Geometry: final body of the model. Coordinates: model frame, mm. A direction names the side the tool comes from. Give positions to 0.01 mm unless a question says otherwise; leave off trailing zeros. Order: outer loops, then holes, each group sorted by start corner. A loop starts at its lowest first (then second) coordinate and runs counter-clockwise, first axis right, second up. Notation, with made-up numbers: (-12.5, 38.5) - (40.5, 38.5) arc R18 cw to (40.5, 64.5) - close; hole circle Ø4 at (48, -35). An arc over 180 degrees is marked (long way). Use one line per item in the form item = value.
from build123d import *

# Parameters (mm, degrees)
F0_R     = 25
F1_DEPTH = 10


# Not quite as in the source:
# - a feature names something its author has since deleted; it is built from what else it names


with BuildPart() as f1:
    # F0 (on Top) → F1 (new body)
    with BuildSketch(Plane.XY):
        with Locations((-0.1409200142, -0.0023476887)):
            Circle(F0_R)
        with BuildLine():
            ThreePointArc((0.7, 23.7306175986), (17.033068856, 16.5380402997), (23.7409395688, 0))
            ThreePointArc((23.7409395688, 0), (23.0200904836, -5.8058286004), (20.9013176879, -11.2590910166))
            ThreePointArc((20.9013176879, -11.2590910166), (20.5602567763, -11.8704697844), (20.2013176879, -12.4715265819))
            ThreePointArc((20.2013176879, -12.4715265819), (0, -23.7409395688), (-20.2013176879, -12.4715265819))
            ThreePointArc((-20.2013176879, -12.4715265819), (-20.5602567763, -11.8704697844), (-20.9013176879, -11.2590910166))
            ThreePointArc((-20.9013176879, -11.2590910166), (-20.5602567763, 11.8704697844), (-0.7, 23.7306175986))
            ThreePointArc((-0.7, 23.7306175986), (0, 23.7409395688), (0.7, 23.7306175986))
        make_face(mode=Mode.SUBTRACT)
        with BuildLine():
            ThreePointArc((5.4607696164, 0), (4.1013743754, 3.6053755749), (0.7, 5.4157183091))
            ThreePointArc((0.7, 5.4157183091), (0.3507241153, 5.4494951508), (0, 5.4607696164))
            ThreePointArc((0, 5.4607696164), (-0.3507241153, 5.4494951508), (-0.7, 5.4157183091))
            ThreePointArc((-0.7, 5.4157183091), (-4.729165212, 2.7303848082), (-5.0401496354, -2.1016413719))
            ThreePointArc((-5.0401496354, -2.1016413719), (-4.8947632961, -2.4210115818), (-4.729165212, -2.7303848082))
            ThreePointArc((-4.729165212, -2.7303848082), (-4.5440391807, -3.028483569), (-4.3401496354, -3.3140769372))
            ThreePointArc((-4.3401496354, -3.3140769372), (0, -5.4607696164), (4.3401496354, -3.3140769372))
            ThreePointArc((4.3401496354, -3.3140769372), (4.5440391807, -3.028483569), (4.729165212, -2.7303848082))
            ThreePointArc((4.729165212, -2.7303848082), (4.8947632961, -2.4210115818), (5.0401496354, -2.1016413719))
            ThreePointArc((5.0401496354, -2.1016413719), (5.354582187, -1.0716596503), (5.4607696164, 0))
        make_face()
        with BuildLine():
            Line((-3.4987264855, 2.0612527399), (0, 2.0612527399))
            Line((0, 2.0612527399), (3.4987264855, 2.0612527399))
            ThreePointArc((3.4987264855, 2.0612527399), (0, -3.5618006487), (-3.4987264855, 2.0612527399))
        make_face(mode=Mode.SUBTRACT)
        with BuildLine():
            Line((-5.0401496354, -2.1016413719), (-20.9013176879, -11.2590910166))
            ThreePointArc((-20.9013176879, -11.2590910166), (-20.5602567763, -11.8704697844), (-20.2013176879, -12.4715265819))
            Line((-20.2013176879, -12.4715265819), (-4.3401496354, -3.3140769372))
            ThreePointArc((-4.3401496354, -3.3140769372), (-4.5440391807, -3.028483569), (-4.729165212, -2.7303848082))
            ThreePointArc((-4.729165212, -2.7303848082), (-4.8947632961, -2.4210115818), (-5.0401496354, -2.1016413719))
        make_face()
        with BuildLine():
            Line((0.7, 5.4157183091), (0.7, 23.7306175986))
            ThreePointArc((0.7, 23.7306175986), (0, 23.7409395688), (-0.7, 23.7306175986))
            Line((-0.7, 23.7306175986), (-0.7, 5.4157183091))
            ThreePointArc((-0.7, 5.4157183091), (-0.3507241153, 5.4494951508), (0, 5.4607696164))
            ThreePointArc((0, 5.4607696164), (0.3507241153, 5.4494951508), (0.7, 5.4157183091))
        make_face()
        with BuildLine():
            ThreePointArc((20.2013176879, -12.4715265819), (20.5602567763, -11.8704697844), (20.9013176879, -11.2590910166))
            Line((20.9013176879, -11.2590910166), (5.0401496354, -2.1016413719))
            ThreePointArc((5.0401496354, -2.1016413719), (4.8947632961, -2.4210115818), (4.729165212, -2.7303848082))
            ThreePointArc((4.729165212, -2.7303848082), (4.5440391807, -3.028483569), (4.3401496354, -3.3140769372))
            Line((4.3401496354, -3.3140769372), (20.2013176879, -12.4715265819))
        make_face()
    extrude(amount=F1_DEPTH)


solid = f1.part
(1) Reachability of faces 1 (the face through (20.39, 12.16, 4.93)), 2 (the face through (0, 4, 10)) from +Z, -Z, +X, -X, +Y, -Y: full face, straight path, thin tool, end or side. Return the list, or none.
Computed values:
face_1 = +Z, -Z
face_2 = +Z, +X, -X, +Y, -Y
(2) Cut plane C-C on y = -14.5. Output: boundary loops of the cut face in (x, z), plus the area to 3 significant figures.
Computed values:
outline = (-20.51, 0) - (-18.8, 0) - (-18.8, 10) - (-20.51, 10) - close; (18.8, 0) - (20.23, 0) - (20.23, 10) - (18.8, 10) - close
area = 31.4 mm²
(3) Cut plane B-B on x = -16. Output: boundary loops of the cut face in (y, z).
Computed values:
outline = (-19.33, 0) - (-17.54, 0) - (-17.54, 10) - (-19.33, 10) - close; (-10.05, 0) - (-8.43, 0) - (-8.43, 10) - (-10.05, 10) - close; (17.54, 0) - (19.32, 0) - (19.32, 10) - (17.54, 10) - close
(4) Cut plane A-A on y = 18. Output: boundary loops of the cut face in (x, z).
Computed values:
outline = (-17.49, 0) - (-15.48, 0) - (-15.48, 10) - (-17.49, 10) - close; (-0.7, 0) - (0.7, 0) - (0.7, 10) - (-0.7, 10) - close; (15.48, 0) - (17.21, 0) - (17.21, 10) - (15.48, 10) - close
(5) Contact query for flat-ended pins moving along their axis: pin 1 Ø3 at (x, z) = (-1, 2.5) entering from +Y; pin 2 Ø3 at (y, z) = (5.5, 7) entering from +X; pin 3 Ø3 at (x, z) = (2, 7) entering from -Y; pin 4 Ø4 at (x, y) = (2, 4) entering from -Z. Output: stop coordinate, or through.
Computed values:
pin_1 = 25
pin_2 = 24.54
pin_3 = -24.99
pin_4 = 0
(6) Pull-direction query (Y, two-part tool) for faces 3 (the face through (-12.382, -7.957, 4.93)), 4 (the face through (-0.07, -5.46, 4.93)), 5 (the face through (11.4, -22.18, 4.93)), 6 (the face through (0, 4, 0)); classes: released by +Y, released by -Y, zero draft, split by the parting line, or undercut.
Computed values:
face_3 = undercut
face_4 = undercut
face_5 = split by the parting line
face_6 = zero draft
(7) Cut plane D-D on z = 2.25. Output: boundary loops of the cut face in (x, y), plus the area to 3 significant figures.
Computed values:
outline = circle Ø50 at (-0.14, 0); hole (-20.9, -11.26) - (-5.04, -2.1) arc R5.46 cw to (-0.7, 5.42) - (-0.7, 23.73) arc R23.74 ccw to start; hole (-20.2, -12.47) arc R23.74 ccw to (20.2, -12.47) - (4.34, -3.31) arc R5.46 cw to (-4.34, -3.31) - close; hole (-3.5, 2.06) arc R3.9 ccw (long way) to (3.5, 2.06) - close; hole (0.7, 5.42) arc R5.46 cw to (5.04, -2.1) - (20.9, -11.26) arc R23.74 ccw to (0.7, 23.73) - close
area = 326 mm²
(8) Ray query, line 1 along Y through (x, z) = (-12.5, 4.25); line 2 along X through (y, z) = (10, 9.75); line 3 along X through (y, z) = (6.5, 9). Return the intervals inside material, ascending.
Computed values:
line_1 = -21.73 to -20.18, -8.03 to -6.41, 20.18 to 21.73
line_2 = -23.05 to -21.53, -0.7 to 0.7, 21.53 to 22.77
line_3 = -24.28 to -22.83, -0.7 to 0.7, 22.83 to 24
